from build123d import *

# Parameters (mm, degrees)
SKETCH4_R            = 19.1
BOSS_EXTRUDE4_DEPTH  = 80
BOSS_EXTRUDE5_START  = 2
BOSS_EXTRUDE5_DEPTH  = 2
SKETCH6_R            = 5
CUT_EXTRUDE1_DEPTH   = 2
BOSS_EXTRUDE7_DEPTH  = 30
SKETCH8_R            = 11
CUT_EXTRUDE2_DEPTH   = 30
SKETCH9_R            = 1.5
CUT_EXTRUDE3_DEPTH   = 30
SKETCH11_W           = 5
SKETCH11_H           = 112
BOSS_EXTRUDE8_DEPTH  = 20
SKETCH12_W           = 5
SKETCH12_H           = 112
BOSS_EXTRUDE9_DEPTH  = 20
SKETCH13_R           = 1.5
CUT_EXTRUDE4_DEPTH   = 20
SKETCH14_R           = 1.5
CUT_EXTRUDE5_DEPTH   = 20
SKETCH16_W           = 30
SKETCH16_H           = 70
BOSS_EXTRUDE10_DEPTH = 30
SKETCH21_W           = 6
SKETCH21_H           = 4.9
CUT_EXTRUDE6_DEPTH   = 70
SKETCH23_W           = 3
SKETCH23_H           = 70
BOSS_EXTRUDE11_DEPTH = 30
FILLET5_R            = 3.2
FILLET6_R            = 20
SKETCH26_W           = 112
SKETCH26_H           = 40
CUT_EXTRUDE10_DEPTH  = 15
SKETCH27_W           = 6.865199721
SKETCH27_H           = 6.850856093
SKETCH27_W_2         = 7.923200186
SKETCH27_H_2         = 5.884780205
CUT_EXTRUDE11_DEPTH  = 131.000961535
SKETCH28_W           = 12.4
SKETCH28_H           = 15
BOSS_EXTRUDE12_DEPTH = 70
FILLET7_R            = 10
SKETCH29_R           = 1.5
CUT_EXTRUDE12_DEPTH  = 129.917648132
SKETCH30_R           = 1.5
CUT_EXTRUDE13_DEPTH  = 15
FILLET8_R            = 10


# Some blends are built 0.0001 mm under size
with BuildPart() as part:
    # Sketch4 → Boss-Extrude4 (new body)
    with BuildSketch(Plane.XY):
        with BuildLine():
            Line((22.5, 0), (22.5, -60))
            Line((22.5, -60), (17.5, -60))
            Line((17.5, -60), (17.5, -40))
            ThreePointArc((17.5, -40), (12.374368671, -27.625631329), (0, -22.5))
            ThreePointArc((0, -22.5), (-22.5, 0), (0, 22.5))
            ThreePointArc((0, 22.5), (12.374368671, 27.625631329), (17.5, 40))
            Line((17.5, 40), (17.5, 60))
            Line((17.5, 60), (22.5, 60))
            Line((22.5, 60), (22.5, 0))
        make_face()
        Circle(SKETCH4_R, mode=Mode.SUBTRACT)
    extrude(amount=BOSS_EXTRUDE4_DEPTH)

    # Sketch5 → Boss-Extrude5 (add)
    with BuildSketch(Plane(origin=(0, 0, 0), x_dir=(-1, 0, 0), z_dir=(0, 0, -1)).offset(BOSS_EXTRUDE5_START)):
        with BuildLine():
            Line((-17.5, 60), (-22.5, 60))
            Line((-22.5, 60), (-22.5, -60))
            Line((-22.5, -60), (-17.5, -60))
            Line((-17.5, -60), (-17.5, -40))
            ThreePointArc((-17.5, -40), (-12.374368671, -27.625631329), (0, -22.5))
            ThreePointArc((0, -22.5), (22.5, 0), (0, 22.5))
            ThreePointArc((0, 22.5), (-12.374368671, 27.625631329), (-17.5, 40))
            Line((-17.5, 40), (-17.5, 60))
        make_face()
    extrude(amount=-BOSS_EXTRUDE5_DEPTH)

    # Sketch6 → Cut-Extrude1 (cut)
    with BuildSketch(Plane(origin=(0, 0, -2), x_dir=(-1, 0, 0), z_dir=(0, 0, -1))):
        Circle(SKETCH6_R)
    extrude(amount=-CUT_EXTRUDE1_DEPTH, mode=Mode.SUBTRACT)

    # Sketch7 → Boss-Extrude7 (add)
    with BuildSketch(Plane.XY.offset(80)):
        with BuildLine():
            Line((17.5, 60), (17.5, 7.652450588))
            ThreePointArc((17.5, 7.652450588), (19.1, 0), (17.5, -7.652450588))
            Line((17.5, -7.652450588), (17.5, -60))
            Line((17.5, -60), (22.5, -60))
            Line((22.5, -60), (22.5, 60))
            Line((22.5, 60), (17.5, 60))
        make_face()
    extrude(amount=BOSS_EXTRUDE7_DEPTH)

    # Sketch8 → Cut-Extrude2 (cut)
    with BuildSketch(Plane(origin=(0, 0, -2), x_dir=(-1, 0, 0), z_dir=(0, 0, -1))):
        Circle(SKETCH8_R)
    extrude(amount=-CUT_EXTRUDE2_DEPTH, mode=Mode.SUBTRACT)

    # Sketch9 → Cut-Extrude3 (cut)
    with BuildSketch(Plane(origin=(0, 0, -2), x_dir=(-1, 0, 0), z_dir=(0, 0, -1))):
        with Locations((0, 13.5)):
            Circle(SKETCH9_R)
        with Locations((13.5, 0)):
            Circle(SKETCH9_R)
        with Locations((0, -13.5)):
            Circle(SKETCH9_R)
        with Locations((-13.5, 0)):
            Circle(SKETCH9_R)
    extrude(amount=-CUT_EXTRUDE3_DEPTH, mode=Mode.SUBTRACT)

    # Sketch11 → Boss-Extrude8 (add)
    with BuildSketch(Plane.XZ.offset(60)):
        with Locations((20, 54)):
            Rectangle(SKETCH11_W, SKETCH11_H)
    extrude(amount=BOSS_EXTRUDE8_DEPTH)

    # Sketch12 → Boss-Extrude9 (add)
    with BuildSketch(Plane(origin=(0, 60, 0), x_dir=(1, 0, 0), z_dir=(0, 1, 0))):
        with Locations((20, -54)):
            Rectangle(SKETCH12_W, SKETCH12_H)
    extrude(amount=BOSS_EXTRUDE9_DEPTH)

    # Sketch13 → Cut-Extrude4 (cut)
    with BuildSketch(Plane.ZY.offset(-17.5)):
        with Locations((26, 60)):
            Circle(SKETCH13_R)
        with Locations((54, 60)):
            Circle(SKETCH13_R)
        with Locations((82, 60)):
            Circle(SKETCH13_R)
        with Locations((82, -60)):
            Circle(SKETCH13_R)
        with Locations((54, -60)):
            Circle(SKETCH13_R)
        with Locations((26, -60)):
            Circle(SKETCH13_R)
    extrude(amount=-CUT_EXTRUDE4_DEPTH, mode=Mode.SUBTRACT)

    # Sketch14 → Cut-Extrude5 (cut)
    with BuildSketch(Plane.ZY.offset(-17.5)):
        with Locations((95, 37.652450588)):
            Circle(SKETCH14_R)
        with Locations((95, -37.652450588)):
            Circle(SKETCH14_R)
    extrude(amount=-CUT_EXTRUDE5_DEPTH, mode=Mode.SUBTRACT)

    # Sketch16 → Boss-Extrude10 (add)
    with BuildSketch(Plane(origin=(22.5, 0, 0), x_dir=(0, 0, -1), z_dir=(1, 0, 0))):
        with Locations((-13, 0)):
            Rectangle(SKETCH16_W, SKETCH16_H)
    extrude(amount=BOSS_EXTRUDE10_DEPTH)

    # Sketch21 → Cut-Extrude6 (cut)
    with BuildSketch(Plane(origin=(0, 35, 0), x_dir=(1, 0, 0), z_dir=(0, 1, 0))):
        Polygon((34.8, -2.9), (27.4, -2.9), (27.4, -10.3), (29.4, -10.3), (29.4, -8.3), (32.4, -10.3), (32.4, -15.7), (29.4, -17.7), (29.4, -15.7), (27.4, -15.7), (27.4, -23.1), (34.9, -23.1), (40.9, -23.1), (47.6, -23.1), (47.6, -15.7), (45.6, -15.7), (45.6, -17.7), (42.6, -15.7), (42.6, -10.3), (45.6, -8.3), (45.6, -10.3), (47.6, -10.3), (47.6, -2.9), (40.2, -2.9), (40.2, -4.9), (42.2, -4.9), (40.2, -7.9), (34.8, -7.9), (32.8, -4.9), (34.8, -4.9), align=None)
        with Locations((37.9, -25.55)):
            Rectangle(SKETCH21_W, SKETCH21_H)
    extrude(amount=-CUT_EXTRUDE6_DEPTH, mode=Mode.SUBTRACT)

    # Sketch23 → Boss-Extrude11 (add)
    with BuildSketch(Plane.XY.offset(28)):
        with Locations((42.4, 0)):
            Rectangle(SKETCH23_W, SKETCH23_H)
        with Locations((24, 0)):
            Rectangle(SKETCH23_W, SKETCH23_H)
        with Locations((33.4, 0)):
            Rectangle(SKETCH23_W, SKETCH23_H)
    extrude(amount=BOSS_EXTRUDE11_DEPTH)

    # Fillet5
    fillet5_edges = [part.edges().sort_by_distance(p)[0] for p in [
        (25.5, 0, 28),
        (31.9, 0, 28),
    ]]
    fillet(fillet5_edges, radius=FILLET5_R - 0.0001)  # a hair under: the kernel refuses the full size

    # Fillet6
    # the kernel refuses this fillet: 20 mm, written as the material it adds along each edge
    with BuildSketch(Plane(origin=(43.9, 35, 28), x_dir=(1, 0, 0), z_dir=(0, -1, 0))) as fillet6_piece_1:
        with BuildLine():
            CenterArc((20, 16.432893841), FILLET6_R, 180, 55.249774246)
            Line((0, 16.432893841), (-0.4, 16.432893841))
            Line((-0.4, 16.432893841), (-0.4, 0))
            Line((-0.4, 0), (0, -0.4))
            ThreePointArc((0, -0.4), (4.3, -0.4), (8.372, -0.328657877))
            Line((8.372, -0.328657877), (8.6, 0))
        make_face()
    extrude(amount=70)

    # Sketch26 → Cut-Extrude10 (cut)
    with BuildSketch(Plane.ZY.offset(-17.5)):
        with Locations((54, -60)):
            Rectangle(SKETCH26_W, SKETCH26_H)
        with Locations((54, 60)):
            Rectangle(SKETCH26_W, SKETCH26_H)
    extrude(amount=-CUT_EXTRUDE10_DEPTH, mode=Mode.SUBTRACT)

    # Sketch27 → Cut-Extrude11 (cut, through all)
    with BuildSketch(Plane(origin=(0, 0, -2), x_dir=(-1, 0, 0), z_dir=(0, 0, -1))):
        with Locations((-19.06740014, 38.425428047)):
            Rectangle(SKETCH27_W, SKETCH27_H)
        with Locations((-18.538399907, -37.942390102)):
            Rectangle(SKETCH27_W_2, SKETCH27_H_2)
    extrude(amount=-CUT_EXTRUDE11_DEPTH, mode=Mode.SUBTRACT)

    # Sketch28 → Boss-Extrude12 (add)
    with BuildSketch(Plane(origin=(0, 35, 0), x_dir=(1, 0, 0), z_dir=(0, 1, 0))):
        with Locations((28.7, -95)):
            Rectangle(SKETCH28_W, SKETCH28_H)
    extrude(amount=-BOSS_EXTRUDE12_DEPTH)

    # Fillet7
    # the kernel refuses this fillet: 10 mm, written as the material it adds along each edge
    with BuildSketch(Plane(origin=(22.5, 35, 102.5), x_dir=(0, 0, 1), z_dir=(0, -1, 0))) as fillet7_piece_1:
        with BuildLine():
            CenterArc((10, -9.682458366), FILLET7_R, 104.477512186, 75.522487814)
            Line((0, -9.682458366), (-0.2, -9.682458366))
            Line((-0.2, -9.682458366), (-0.2, 0))
            Line((-0.2, 0), (0, 0.2))
            ThreePointArc((0, 0.2), (3.75, 0.2), (7.45, 0.193649167))
            Line((7.45, 0.193649167), (7.5, 0))
        make_face()
    extrude(amount=70)
    with BuildSketch(Plane(origin=(22.5, 35, 87.5), x_dir=(0, 0, -1), z_dir=(0, -1, 0))) as fillet7_piece_2:
        with BuildLine():
            CenterArc((FILLET7_R, FILLET7_R), FILLET7_R, 180, 90)
            Line((0, FILLET7_R), (-FILLET7_R * 0.02, FILLET7_R))
            Line((-FILLET7_R * 0.02, FILLET7_R), (-FILLET7_R * 0.02, -FILLET7_R * 0.02))
            Line((-FILLET7_R * 0.02, -FILLET7_R * 0.02), (FILLET7_R, -FILLET7_R * 0.02))
            Line((FILLET7_R, -FILLET7_R * 0.02), (FILLET7_R, 0))
        make_face()
    extrude(amount=70)

    # Sketch29 → Cut-Extrude12 (cut, through all)
    with BuildSketch(Plane(origin=(34.9, 0, 0), x_dir=(0, 0, -1), z_dir=(1, 0, 0))):
        with Locations((-95, 25)):
            Circle(SKETCH29_R)
        with Locations((-95, -25)):
            Circle(SKETCH29_R)
    extrude(amount=-CUT_EXTRUDE12_DEPTH, mode=Mode.SUBTRACT)

    # Sketch30 → Cut-Extrude13 (cut)
    with BuildSketch(Plane(origin=(43.9, 0, 0), x_dir=(0, 0, -1), z_dir=(1, 0, 0))):
        with Locations(Location((-51.216446921, 25, 0), (0, 0, 90))):
            Circle(SKETCH30_R)
        with Locations(Location((-51.216446921, -25, 0), (0, 0, 90))):
            Circle(SKETCH30_R)
    extrude(amount=-CUT_EXTRUDE13_DEPTH, mode=Mode.SUBTRACT)

    # Fillet8
    # the kernel refuses this fillet: 10 mm, written as the material it adds along each edge
    with BuildSketch(Plane(origin=(22.5, -35, 58), x_dir=(0, 0, 1), z_dir=(0, 1, 0))) as fillet8_piece_1:
        with BuildLine():
            CenterArc((7.141428429, 10), FILLET8_R, 224.427004001, 45.572995999)
            Line((0, 3), (-0.142828569, 2.86))
            ThreePointArc((-0.142828569, 2.86), (-0.2, 1.5), (-0.2, 0))
            Line((-0.2, 0), (0, -0.2))
            Line((0, -0.2), (7.141428429, -0.2))
            Line((7.141428429, -0.2), (7.141428429, 0))
        make_face()
    extrude(amount=70)


solid = part.part
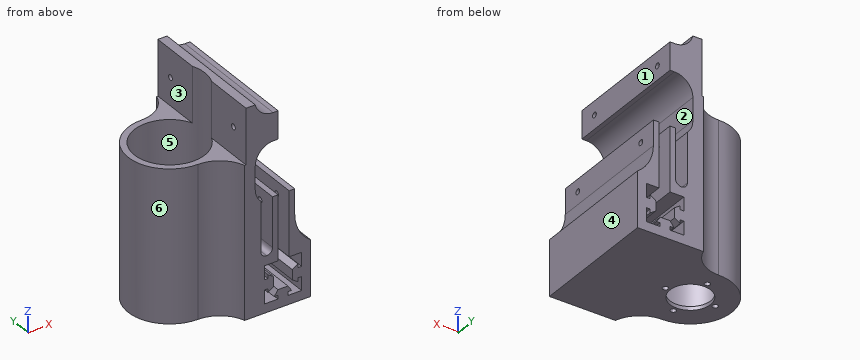
Source: CAD feature listing. Evaluate the final solid. Frame: model axes, mm. Face numbers are marked on the shaded views. A direction names the side the tool comes from. Coordinates: 2 decimals unless noted, no trailing zeros. Order: outer loops, then holes, each group sorted by start corner. A loop starts at its lowest first (then second) coordinate and runs counter-clockwise, first axis right, second up.
Item 1: Set-up query: the marked faces 1, 2 and 3. Return all of +Z, -Z, +X, -X, +Y, -Y with unobstructed straight access to the full face (end or side cutting, diameter ignored); none if empty.
Output values:
face 1: +Z, +X, +Y, -Y
face 2: +X, +Y, -Y
face 3: +Z, -X, +Y, -Y
Item 2: Cut plane D-D (y = 0). Count the separate pieces of the cut face and the enclosed holes in it, plus the area to 3 significant figures.
Output values:
separate pieces: 4
enclosed holes: 0
area: 1,790 mm2
Item 3: First-contact query: P1, Ø1.5, axis at x = 31.5, y = 2.5, coming from the +Z side; P2, Ø1, axis at y = 0, z = 9.5, coming from the -X side; P3, Ø12, axis at y = 16, z = 68, coming from the +X side; P4, Ø10, axis at x = 38, z = 79.5, coming from the -Y side. Flat tips, straight axial feed; report the tip coordinate or a pass-through.
Output values:
P1: stops at z = 102.6
P2: stops at x = -22.5
P3: stops at x = 23.01
P4: passes through
Item 4: Material intervals for line 1 (Y direction, x = 26.25, z = 95); line 2 (X direction, y = 0, z = 23); line 3 (Z direction, x = 30, y = 26), sorted ascending.
Output values:
line 1: y = -35 to -26.5, -23.5 to 23.5, 26.5 to 35
line 2: x = -22.5 to -19.1, 19.1 to 27.4, 47.6 to 52.5
line 3: z = -2 to 2.9, 8.7 to 17.3, 23.1 to 28.28, 87.18 to 93.88, 96.12 to 102.74
Item 5: Cut plane B-B (z = 95). Return loops of the section in (x, y).
Output values:
outline: (17.5, -35) - (34.9, -35) - (34.9, -26.5) - (17.5, -26.5) - close; (17.5, -23.5) - (34.9, -23.5) - (34.9, 23.5) - (17.5, 23.5) - (17.5, 7.65) arc R19.1 cw to (17.5, -7.65) - close; (17.5, 26.5) - (34.9, 26.5) - (34.9, 35) - (17.5, 35) - close
Item 6: Pull-direction query (X, two-part tool) for the marked faces 4, 5 and 6; classes: pulls with the +X half, pulls with the -X half, needs draft (parallel to the pull), parting line crosses it, or undercut.
Output values:
face 4: pulls with the +X half
face 5: undercut
face 6: pulls with the -X half
Item 7: Cut plane A-A (z = 46). Return loops of the section in (x, y).
Output values:
outline: (0, -22.5) arc R17.5 cw to (16.77, -35) - (25.5, -35) - (25.5, 35) - (16.77, 35) arc R17.5 cw to (0, 22.5) arc R22.5 ccw to start; (31.9, -35) - (34.9, -35) - (34.9, 35) - (31.9, 35) - close; (40.9, -35) - (43.9, -35) - (43.9, 35) - (40.9, 35) - close; hole circle Ø38.2 at (0, 0)
Item 8: Cut plane C-C (x = 13.5). Return loops of the section in (y, z), plus the area to 3 significant figures.
Output values:
outline: (-28.86, -2) - (-1.5, -2) - (-1.5, 0) - (-13.51, 0) - (-13.51, 80) - (-28.86, 80) - close; (1.5, -2) - (28.86, -2) - (28.86, 80) - (13.51, 80) - (13.51, 0) - (1.5, 0) - close
area: 2,570 mm2
